Part print with two shaded views. Sizes in mm from the minimum x, y, z corner. Give positions to 0.01 mm unless a question says otherwise; leave off trailing zeros. Write each loop counter-clockwise with the first axis right and the second up, starting at its lowest first coordinate (ties: lowest second). Pieces come first, ordered by that corner, then holes.
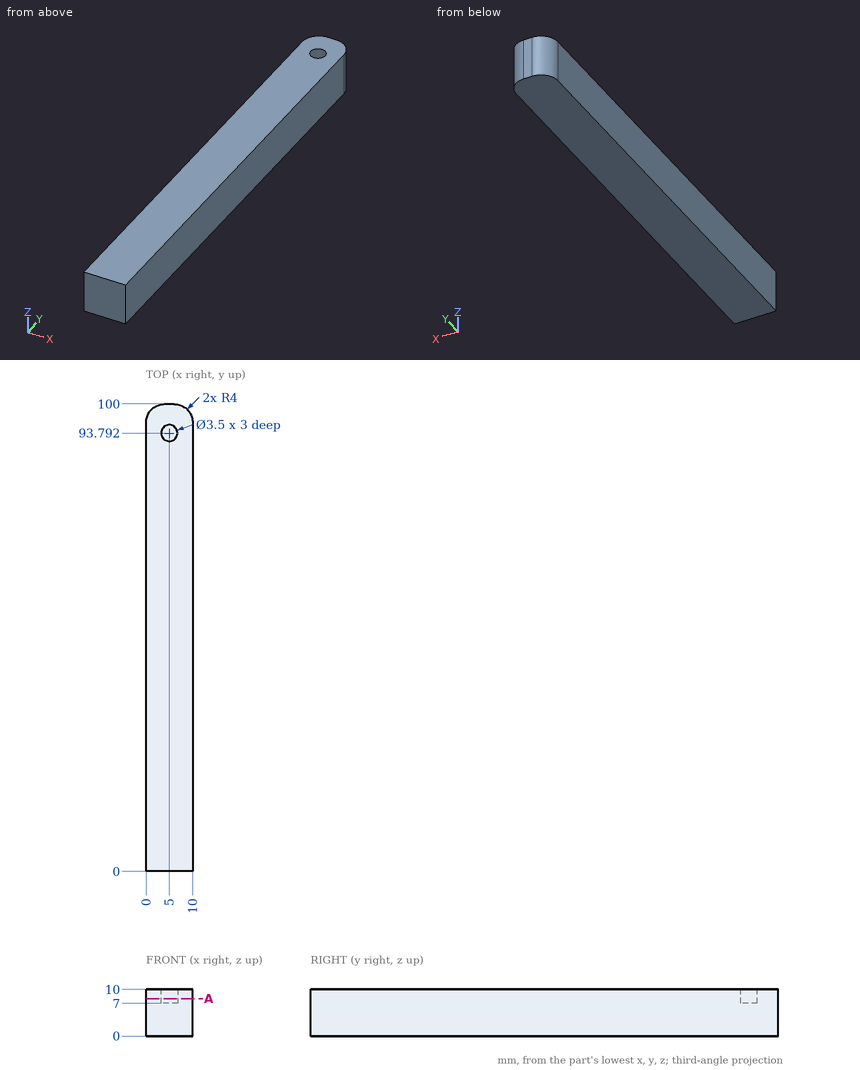
1) Pin check, flat tip, straight feed: pin 1 Ø1 at (x, y) = (4.5, 94.5) entering from +Z. Stop position of the tip, or through.
Answers follow:
pin 1: stops at z = 7
2) Wall check: L1, parallel to Y at x = 5, z = 8.05; L2, parallel to Y at x = 3.75, z = 6.25; L3, parallel to Y at x = 2.5, z = 7. Give the ranges that are in metal, low to high.
Answers follow:
L1: y = 0 to 92.04, 95.54 to 100
L2: y = 0 to 99.99
L3: y = 0 to 99.71
3) Saw through at A-A, the plane z = 8. Write the cut outline in (x, y).
Answers follow:
outline: (0, 0) - (10, 0) - (10, 96) arc R4 ccw to (6, 100) - (4, 100) arc R4 ccw to (0, 96) - close; hole circle Ø3.5 at (5, 93.79)
